Design review of the part built by this model. Coordinates are the model's own, in mm. A direction names the side the tool comes from. Give positions to 0.01 mm unless a question says otherwise; leave off trailing zeros. Order: outer loops, then holes, each group sorted by start corner. A loop starts at its lowest first (then second) coordinate and runs counter-clockwise, first axis right, second up. Notation, with made-up numbers: (27.5, 9.5) -> (73.5, 9.5) arc R7 ccw to (73.5, 13.5) -> close; hole circle Ø3 at (-11, 80). An arc over 180 degrees is marked (long way). One line per item, written item: value.
from build123d import *

# Parameters (mm, degrees)
SKETCH1_R           = 25
BOSS_EXTRUDE1_DEPTH = 4
SKETCH2_R           = 7
SKETCH2_R_2         = 5
BOSS_EXTRUDE2_DEPTH = 24
SKETCH3_R           = 1.5
CUT_EXTRUDE1_DEPTH  = 24


with BuildPart() as part:
    # Sketch1 → Boss-Extrude1 (new body)
    with BuildSketch(Plane.XY):
        Circle(SKETCH1_R)
    extrude(amount=BOSS_EXTRUDE1_DEPTH)

    # Sketch2 → Boss-Extrude2 (add)
    with BuildSketch(Plane.XY.offset(4)):
        Circle(SKETCH2_R)
        Circle(SKETCH2_R_2, mode=Mode.SUBTRACT)
    extrude(amount=BOSS_EXTRUDE2_DEPTH)

    # Sketch3 → Cut-Extrude1 (cut)
    with BuildSketch(Plane(origin=(0, 0, 0), x_dir=(-1, 0, 0), z_dir=(0, 0, -1))):
        with Locations((0, 14)):
            Circle(SKETCH3_R)
        with Locations((12.124355653, 7)):
            Circle(SKETCH3_R)
        with Locations((12.124355653, -7)):
            Circle(SKETCH3_R)
        with Locations((0, -14)):
            Circle(SKETCH3_R)
        with Locations((-12.124355653, -7)):
            Circle(SKETCH3_R)
        with Locations((-12.124355653, 7)):
            Circle(SKETCH3_R)
    extrude(amount=-CUT_EXTRUDE1_DEPTH, mode=Mode.SUBTRACT)


solid = part.part
Item 1: Add section B-B on y = -14. Give the boundary of the cut face in (x, z).
Returned:
outline: (-20.71, 0) -> (-1.5, 0) -> (-1.5, 4) -> (-20.71, 4) -> close; (1.5, 0) -> (20.71, 0) -> (20.71, 4) -> (1.5, 4) -> close
Item 2: Clearance check with flat-ended pins moving along their axes: P1, Ø12, axis at y = -9.5, z = 16, coming from the -X side; P2, Ø3.5, axis at x = 0, y = -14, coming from the +Z side; P3, Ø1, axis at x = 5, z = 10, coming from the +Y side. State where each tip first meets the part, or that it passes through.
Returned:
P1: x = -6.06
P2: z = 4
P3: y = 5.36
Item 3: Machinability: for faces 5 (the flat face through (5.2, -5.2, 4)), 6 (the cylindrical face through (11.43, 5.67, 1.97)), which of the approach directions +Z, -Z, +X, -X, +Y, -Y give a long, thin tool a straight path to every point of the face, cutting with its end or side? Answer none if there is none.
Returned:
face 5: +Z
face 6: +Z, -Z
Item 4: To check wall thickness, follow line 1 along Y through (x, z) = (0, 2.8); line 2 along Z through (x, y) = (2, 12); line 3 along Y through (x, z) = (0, 23). State the ranges of each line that lie inside material, in increasing order. Write a range as from..to.
Returned:
line 1: -25..-15.5, -12.5..12.5, 15.5..25
line 2: 0..4
line 3: -7..-5, 5..7
Item 5: Add section A-A on x = 0. Give the boundary of the cut face in (y, z).
Returned:
outline: (-25, 0) -> (-15.5, 0) -> (-15.5, 4) -> (-25, 4) -> close; (-12.5, 0) -> (12.5, 0) -> (12.5, 4) -> (7, 4) -> (7, 28) -> (5, 28) -> (5, 4) -> (-5, 4) -> (-5, 28) -> (-7, 28) -> (-7, 4) -> (-12.5, 4) -> close; (15.5, 0) -> (25, 0) -> (25, 4) -> (15.5, 4) -> close
Item 6: Draft analysis for pull direction X (two halves, no side actions). For faces 1 (the cylindrical face through (6.466, -2.681, 15.832)), 2 (the cylindrical face through (-1.08, -4.88, 15.83)), 3 (the flat face through (0, 0, 4)), 4 (the flat face through (0, 0, 0)), state which applies: pulls with the +X half, pulls with the -X half, needs draft (parallel to the pull), parting line crosses it, or undercut.
Returned:
face 1: parting line crosses it
face 2: undercut
face 3: undercut
face 4: needs draft
Item 7: Add section D-D on x = 16.5. Give the boundary of the cut face in (y, z).
Returned:
outline: (-18.78, 0) -> (18.78, 0) -> (18.78, 4) -> (-18.78, 4) -> close
Item 8: Add section C-C on z = 23. Give the boundary of the cut face in (x, y).
Returned:
outline: circle Ø14 at (0, 0); hole circle Ø10 at (0, 0)
